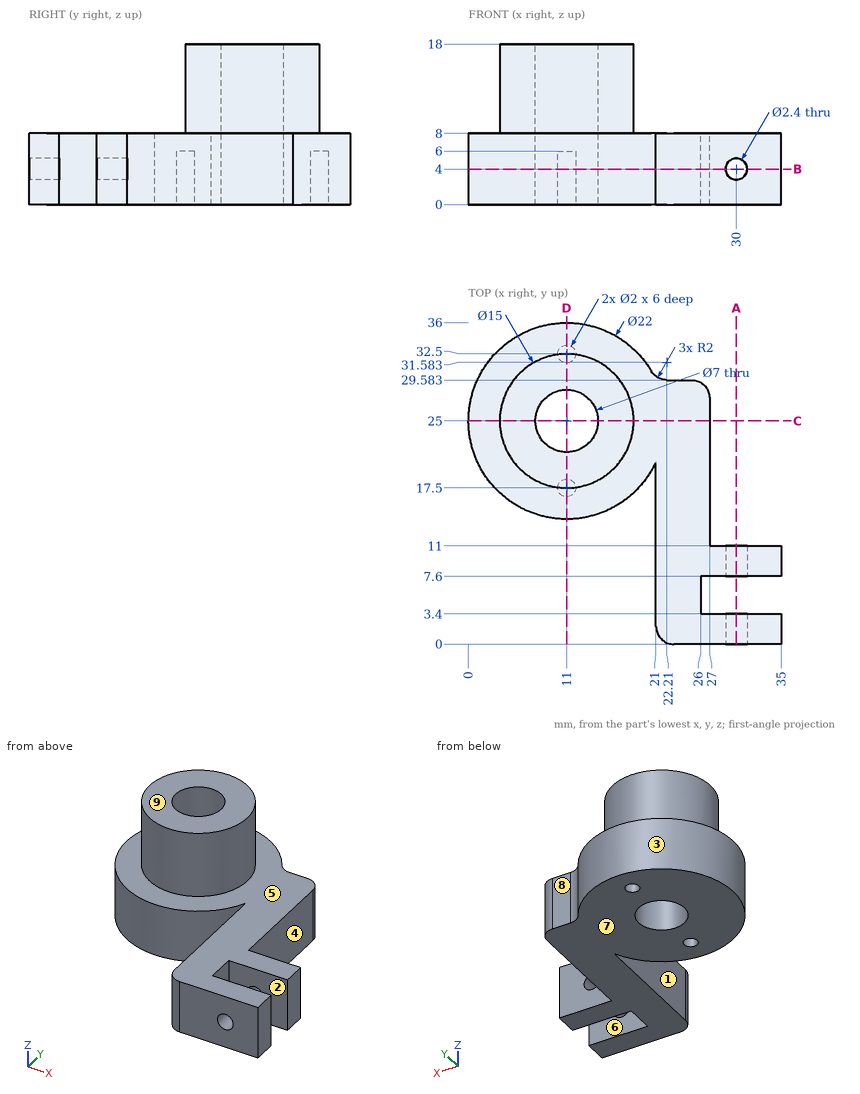
For this review, use the dimensioned drawing (mm, ordinates from the lowest corner) and the shaded views. A direction names the side the tool comes from. Round coordinates to 2 decimals unless told otherwise and drop trailing zeros. Write each loop counter-clockwise with the first axis right and the second up, starting at its lowest first coordinate (ties: lowest second). Pieces come first, ordered by that corner, then holes. Notation, with made-up numbers: (-6, 36.5) - (44, 36.5) arc R23 cw to (44, 73.5) - close; hole circle Ø1 at (-33, 74.5). An arc over 180 degrees is marked (long way). Use a Markdown table: item, result.
Q1. Machinability: for the marked faces 5, 6, 7, 8 and 9, which of the approach directions +Z, -Z, +X, -X, +Y, -Y give a long, thin tool a straight path to every point of the face, cutting with its end or side? Answer none if there is none.
Derived:
| item | result |
|---|---|
| face 5 | +Z |
| face 6 | +Z, -Z, +X |
| face 7 | -Z, +X, -X, +Y, -Y |
| face 8 | +Z, -Z, +X, +Y |
| face 9 | +Z, +X, -X, +Y, -Y |
Q2. Clearance check with flat-ended pins moving along their axes: pin 1 (0.8 mm diameter, centred on x = 24, z = 2.5, fed in from +Y); pin 2 (9 mm diameter, centred on y = 14.5, z = 3.5, fed in from -X); pin 3 (9 mm diameter, centred on x = 31, z = 2, fed in from +Y) (1 decimal); pin 4 (2 mm diameter, centred on x = 30, z = 4, fed in from -Y). State where each tip first meets the part, or that it passes through.
Derived:
| item | result |
|---|---|
| pin 1 | stops at y = 29.58 |
| pin 2 | stops at x = 1.78 |
| pin 3 | stops at y = 28.9 |
| pin 4 | passes through |
Q3. We need section B-B (z = 4). Give the boundary of the cut face in (x, y) (1 decimal), plus the area to 3 significant figures.
Derived:
| item | result |
|---|---|
| outline | (20.5, 30.6) arc R11 ccw (long way) to (21, 20.4) - (21, 2) arc R2 ccw to (23, 0) - (28.8, 0) - (28.8, 3.4) - (26, 3.4) - (26, 7.6) - (28.8, 7.6) - (28.8, 11) - (27, 11) - (27, 27.6) arc R2 ccw to (25, 29.6) - (22.2, 29.6) arc R2 cw to start; (31.2, 0) - (35, 0) - (35, 3.4) - (31.2, 3.4) - close; (31.2, 7.6) - (35, 7.6) - (35, 11) - (31.2, 11) - close; hole circle Ø7 at (11, 25); hole circle Ø2 at (11, 17.5); hole circle Ø2 at (11, 32.5) |
| area | 539 mm2 |
Q4. We need section C-C (y = 25). Give the boundary of the cut face in (x, z).
Derived:
| item | result |
|---|---|
| outline | (0, 0) - (7.5, 0) - (7.5, 18) - (3.5, 18) - (3.5, 8) - (0, 8) - close; (14.5, 0) - (27, 0) - (27, 8) - (18.5, 8) - (18.5, 18) - (14.5, 18) - close |
Q5. We need section D-D (x = 11). Give the boundary of the cut face in (y, z).
Derived:
| item | result |
|---|---|
| outline | (14, 0) - (16.5, 0) - (16.5, 6) - (18.5, 6) - (18.5, 0) - (21.5, 0) - (21.5, 18) - (17.5, 18) - (17.5, 8) - (14, 8) - close; (28.5, 0) - (31.5, 0) - (31.5, 6) - (33.5, 6) - (33.5, 0) - (36, 0) - (36, 8) - (32.5, 8) - (32.5, 18) - (28.5, 18) - close |
Q6. Wall thickness on line 1 along Y through (x, z) = (11, 2.75); line 2 along X through (y, z) = (2, 4); line 3 along Z through (x, y) = (16.5, 34): over which ranges is each line inside the solid? List them lowest first.
Derived:
| item | result |
|---|---|
| line 1 | y = 14 to 16.5, 18.5 to 21.5, 28.5 to 31.5, 33.5 to 36 |
| line 2 | x = 21 to 28.8, 31.2 to 35 |
| line 3 | z = 0 to 8 |
Q7. The part is to be moulded in two halves that separate along X. For the marked faces 1, 2, 3 and 4, say which applies: pulls with the +X half, pulls with the -X half, needs draft (parallel to the pull), parting line crosses it, or undercut.
Derived:
| item | result |
|---|---|
| face 1 | undercut |
| face 2 | needs draft |
| face 3 | undercut |
| face 4 | pulls with the +X half |
Q8. We need section A-A (x = 30). Give the boundary of the cut face in (y, z).
Derived:
| item | result |
|---|---|
| outline | (0, 0) - (3.4, 0) - (3.4, 2.8) - (0, 2.8) - close; (0, 5.2) - (3.4, 5.2) - (3.4, 8) - (0, 8) - close; (7.6, 0) - (11, 0) - (11, 2.8) - (7.6, 2.8) - close; (7.6, 5.2) - (11, 5.2) - (11, 8) - (7.6, 8) - close |
